Work out the finished part from the listing and answer in its coordinate system (mm). A direction names the side the tool comes from. Give positions to 0.01 mm unless a question says otherwise; leave off trailing zeros. Order: outer loops, then holes, each group sorted by start corner. A loop starts at its lowest first (then second) coordinate and runs counter-clockwise, first axis right, second up. Notation, with made-up numbers: M 84,-12 L 114,-12 A21 cw 114,18 Z; hole C 18,-28 d4. An arc over 180 degrees is marked long. One line per item, written item: value.
Solid Edge part; units mm, degrees
sketch "Sketch1" plane through (0, 0, 0) normal (0, -1, 0) x (1, 0, 0)
  line L0 (1.6, 0) -> (1.6, 2)
  line L1 (1.6, 2) -> (3, 2)
  line L2 (3, 2) -> (3, 4.5)
  line L3 (3, 4.5) -> (4.5, 4.5)
  line L4 (4.5, 4.5) -> (4.5, 2)
  line L5 (4.5, 2) -> (10, 2)
  line L6 (10, 2) -> (10, 0)
  line L7 (10, 0) -> (1.6, 0)
revolve "RevolvedProtrusion1" add sketch "Sketch1" angle 360 about axis through (0, 0, 54) along (0, 0, -1)
hole "Hole_1" at (7, 0, 2) direction (0, 0, -1) diameter 2.459 depth 30 tip angle 118 thread major 3 thread length 2
hole "Hole1" at (0, 7, 2) direction (0, 0, -1) diameter 2.459 depth 30 tip angle 118 thread major 3 thread length 2
hole "Hole2" at (-7, 0, 2) direction (0, 0, -1) diameter 2.459 depth 30 tip angle 118 thread major 3 thread length 2
hole "Hole3" at (0, -7, 2) direction (0, 0, -1) diameter 2.459 depth 30 tip angle 118 thread major 3 thread length 2
properties material "Aluminum, 1060"
(1) Given P1, Ø2, axis at y = -2, z = 1, coming from the +X side; P2, Ø1.5, axis at y = 4.5, z = 1.5, coming from the +X side; P3, Ø4, axis at x = -7, y = 0, coming from the +Z side; P4, Ø1.5, axis at x = 0, y = -7, coming from the +Z side, each flat-ended and moving along its own axis, determine where each tip first touches the part or whether it passes through.
Findings:
P1: stops at x = 9.95
P2: stops at x = 9.27
P3: stops at z = 2
P4: passes through
(2) Section C-C, the plane z = 0.5 is taken. Give the vertices of the cut face in (x, y), then the cut area to 3 significant figures.
Findings:
outline: C 0,0 d20; hole C -7,0 d2.46; hole C 0,0 d3.2; hole C 0,-7 d2.46; hole C 0,7 d2.46; hole C 7,0 d2.46
area: 287 mm^2
(3) Determine the mould class of faces 1 (the cylindrical face through (-2.17, 9.76, 0.99)), 2 (the cylindrical face through (-3, 0, 3)), 3 (the flat face through (2, 0, 0)) for opening direction Y: pulls with the +Y half, pulls with the -Y half, needs draft (parallel to the pull), parting line crosses it, or undercut.
Findings:
face 1: parting line crosses it
face 2: undercut
face 3: needs draft
(4) Section D-D, the plane y = -7 is taken. Give the vertices of the cut face in (x, z).
Findings:
outline: M -7.14,0 L -1.23,0 L -1.23,2 L -7.14,2 Z; M 1.23,0 L 7.14,0 L 7.14,2 L 1.23,2 Z
(5) Which of the six approach directions +Z, -Z, +X, -X, +Y, -Y give full straight-line access (tool end or side, diameter ignored) to faces 4 (the flat face through (4.3, 2.1, 2)), 5 (the cylindrical face through (-5.8, 0.27, 0.99))?
Findings:
face 4: +Z
face 5: +Z, -Z
(6) Find the intervals of material crossed by probe 1 along Y at (x, z) = (0, 0.5); probe 2 along X at (y, z) = (0, 3.4), in increasing order. Write a range as from..to.
Findings:
probe 1: y = -10..-8.23, -5.77..-1.6, 1.6..5.77, 8.23..10
probe 2: x = -4.5..-3, 3..4.5
(7) Section A-A, the plane x = 0 is taken. Give the vertices of the cut face in (y, z), then the cut area to 3 significant figures.
Findings:
outline: M -10,0 L -8.23,0 L -8.23,2 L -10,2 Z; M -5.77,0 L -1.6,0 L -1.6,2 L -3,2 L -3,4.5 L -4.5,4.5 L -4.5,2 L -5.77,2 Z; M 1.6,0 L 5.77,0 L 5.77,2 L 4.5,2 L 4.5,4.5 L 3,4.5 L 3,2 L 1.6,2 Z; M 8.23,0 L 10,0 L 10,2 L 8.23,2 Z
area: 31.3 mm^2
(8) Section B-B, the plane x = -7.5 is taken. Give the vertices of the cut face in (y, z), then the cut area to 3 significant figures.
Findings:
outline: M -6.61,0 L -1.12,0 L -1.12,2 L -6.61,2 Z; M 1.12,0 L 6.61,0 L 6.61,2 L 1.12,2 Z
area: 22.0 mm^2
